```python
from build123d import *

# Parameters (mm, degrees)
F2_R          = 5.08
F3_W          = 2.3605417221
F3_H          = 1.905
F3_W_2        = 1.651
F3_H_2        = 3.81
F4_DEPTH      = 2.54
F4_DEPTH_BACK = 2.54


with BuildPart() as f1:
    # F0 (on Front) → F1 (revolve)
    with BuildSketch(Plane.XZ):
        with BuildLine():
            Line((0, 50.8), (0, 0))
            Line((0, 0), (19.05, 0))
            Line((19.05, 0), (19.05, 12.7))
            add(Edge.make_bspline(
                [(19.05, 12.7), (14.6501975513, 14.6853360604), (6.1281189575, 18.5307791547), (6.6413755909, 31.399715349), (5.422508764, 39.255582621), (11.7317588055, 42.4059519263), (15.1685345918, 44.1220216453)],
                knots=[0, 0, 0, 0, 0.2826478816, 0.547467185, 0.7534962459, 1, 1, 1, 1], degree=3))
            Line((15.1685345918, 44.1220216453), (15.1685345918, 50.8))
            Line((15.1685345918, 50.8), (0, 50.8))
        make_face()
    revolve(axis=Axis((0, 0, 25.4), (0, 0, -1)))

    # F2
    f2_edges = [f1.edges().sort_by_distance(p)[0] for p in [
        (-19.05, 0, 12.7),
        (-15.168535, 0, 44.122022),
    ]]
    fillet(f2_edges, radius=F2_R)

    # F3 (on Right) → F4 (join, two sides)
    with BuildSketch(Plane.YZ) as f4_sk:
        with Locations((2.005770861, 55.5625)):
            Rectangle(F3_W, F3_H)
        with Locations((0, 55.5625)):
            Rectangle(F3_W_2, F3_H)
        with Locations((-2.005770861, 55.5625)):
            Rectangle(F3_W, F3_H)
        with Locations((0, 58.42)):
            Rectangle(F3_W_2, F3_H_2)
        with Locations((0, 52.705)):
            Rectangle(F3_W_2, F3_H_2)
    extrude(amount=F4_DEPTH)
    extrude(f4_sk.sketch, amount=-F4_DEPTH_BACK)


solid = f1.part
```
Here's how the part is built. I have some questions about the finished solid (model axes, mm). A direction names the side the tool comes from. Coordinates: 2 decimals unless noted, no trailing zeros. Use a Markdown table: item, result. Add a question column.
(1) Please list where these lines run through material, in increasing order: line 1 (X direction, y = -0.5, z = 54); line 2 (Y direction, x = 15, z = 9); line 3 (X direction, y = 5.5, z = 44).
(2) We'd pull the mould along Z, two halves only. Please class faces 6 (the flat face through (0, 0.826, 53)), 7 (the flat face through (0, 3.186, 56)), 8 (the flat face through (0, 2, 56.515)): +Z half, -Z half, draft (parallel to the pull), parting line (faces both ways), or undercut.
(3) For faces 1 (the flat face through (0, -3.186, 56)), 2 (the flat face through (0, -0.826, 53)), 3 (the flat face through (-2.54, 0, 56)), 4 (the cylindrical face through (-15.154, -0.667, 49.041)), 5 (the flat face through (0, 0.826, 58)), which set-ups out of +Z, -Z, +X, -X, +Y, -Y let a thin tool reach every point of the face, with its end or its side?
(4) I'm going to push flat-ended pins straight in: P1, Ø7, axis at y = -1, z = 57, coming from the -X side; P2, Ø3, axis at y = -3, z = 46.5, coming from the +X side; P3, Ø4, axis at x = 0.5, z = 59, coming from the -Y side; P4, Ø10, axis at y = 13, z = 26.5, coming from the +X side. Where does each tip first touch, or does it pass through?
Outcome:
| question | item | result |
|---|---|---|
| 1 | line 1 | x = -2.54 to 2.54 |
| 1 | line 2 | y = -11.74 to 11.74 |
| 1 | line 3 | x = -12.88 to 12.88 |
| 2 | face 6 | undercut |
| 2 | face 7 | draft |
| 2 | face 8 | +Z half |
| 3 | face 1 | +Z, +X, -X, -Y |
| 3 | face 2 | +X, -X, -Y |
| 3 | face 3 | +Z, -X, +Y, -Y |
| 3 | face 4 | +Z |
| 3 | face 5 | +Z, +X, -X, +Y |
| 4 | P1 | stops at x = -2.54 |
| 4 | P2 | stops at x = 15.08 |
| 4 | P3 | stops at y = -0.83 |
| 4 | P4 | passes through |
